Design review of the part shown in the three views and the two pictorial views. Dimensions are in mm from the part's minimum x, y and z. A direction names the side the tool comes from. Round coordinates to 2 decimals unless told otherwise and drop trailing zeros. Write each loop counter-clockwise with the first axis right and the second up, starting at its lowest first coordinate (ties: lowest second). Pieces come first, ordered by that corner, then holes. Notation, with made-up numbers: (60.5, -39.75) -> (119.5, -39.75) arc R9 ccw to (119.5, -33.75) -> close; hole circle Ø11 at (86.25, 29). An arc over 180 degrees is marked (long way). Return JSON: item names as keys, results as strings. Group by question number.
1. Mouldability with a two-part tool opening along Z and no side actions: class the marked faces 1, 2, 3 and 4 as pulls with the +Z half, pulls with the -Z half, needs draft (parallel to the pull), parting line crosses it, or undercut.
2. Take a section at A-A, the plane y = 5. Write out the cut boundary in (x, z).
3. For line 1 along X through (y, z) = (30, 15.25); line 2 along Z through (x, y) = (6.75, 30); line 3 along Y through (x, z) = (18.5, 11), list the stretches that pass through material, from the lowest coordinate up. Write a range as from..to.
4. Take a section at C-C, the plane z = 12.5. Write out the cut boundary in (x, y).
5. Take a section at D-D, the plane x = 33. Write out the cut boundary in (y, z).
6. Tool access review of the marked faces 5, 6, 7 and 8: name each direction out of +Z, -Z, +X, -X, +Y, -Y from which nothing blocks a thin tool from reaching the whole face with its end or side.
7. Take a section at B-B, the plane y = 30. Write out the cut boundary in (x, z).
8. Clearance check with flat-ended pins moving along their axes: P1, Ø5.5, axis at y = 30, z = 12.5, coming from the -X side; P2, Ø5, axis at y = 53.5, z = 11, coming from the -X side; P3, Ø2, axis at x = 58, z = 9.5, coming from the -Y side. State where each tip first meets the part, or that it passes through.
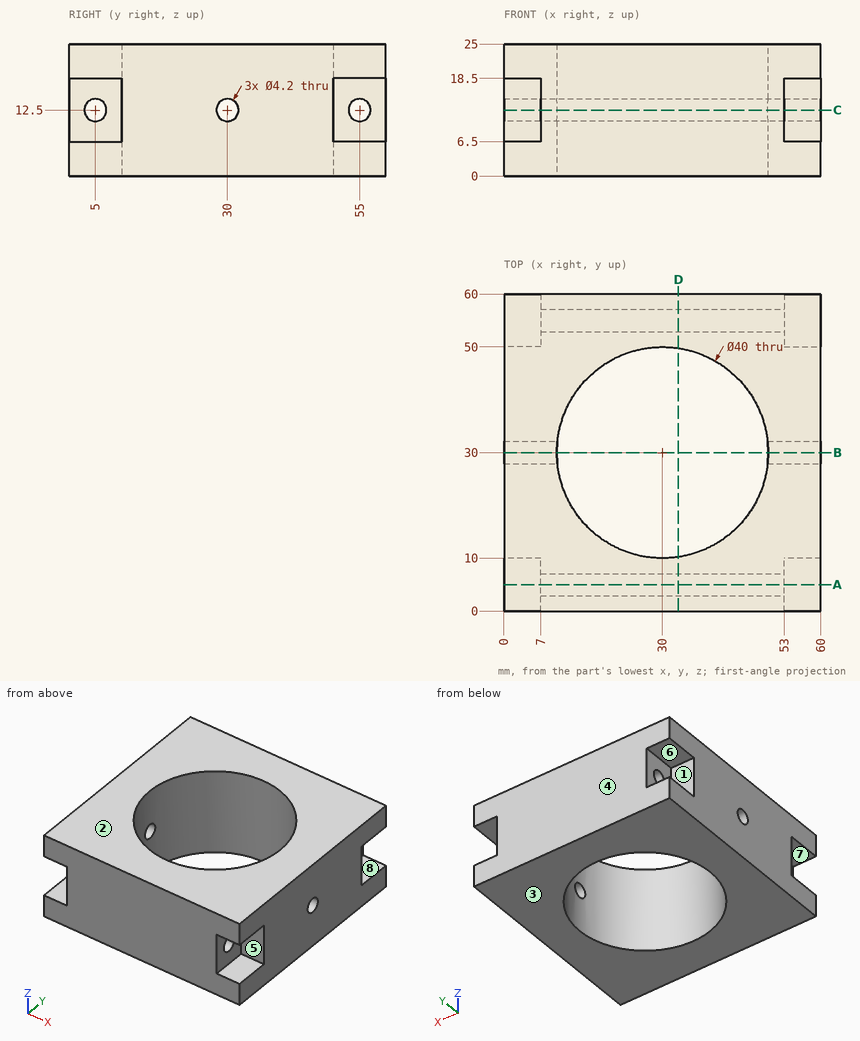
Output:
{
 "1": {"face 1": "undercut", "face 2": "pulls with the +Z half", "face 3": "pulls with the -Z half", "face 4": "needs draft"},
 "2": {"outline": "(0, 0) -> (60, 0) -> (60, 6.5) -> (53, 6.5) -> (53, 10.4) -> (7, 10.4) -> (7, 6.5) -> (0, 6.5) -> close; (0, 18.5) -> (7, 18.5) -> (7, 14.6) -> (53, 14.6) -> (53, 18.5) -> (60, 18.5) -> (60, 25) -> (0, 25) -> close"},
 "3": {"line 1": "x = 0..10, 50..60", "line 2": "z = 0..10.4, 14.6..25", "line 3": "y = 0..3.53, 6.47..13.64, 46.36..53.53, 56.47..60"},
 "4": {"outline": "(0, 10) -> (7, 10) -> (7, 7.1) -> (53, 7.1) -> (53, 10) -> (60, 10) -> (60, 27.9) -> (49.89, 27.9) arc R20 cw to (10.11, 27.9) -> (0, 27.9) -> close; (0, 32.1) -> (10.11, 32.1) arc R20 cw to (49.89, 32.1) -> (60, 32.1) -> (60, 50) -> (53, 50) -> (53, 52.9) -> (7, 52.9) -> (7, 50) -> (0, 50) -> close; (7, 0) -> (53, 0) -> (53, 2.9) -> (7, 2.9) -> close; (7, 57.1) -> (53, 57.1) -> (53, 60) -> (7, 60) -> close"},
 "5": {"outline": "(0, 0) -> (10.23, 0) -> (10.23, 25) -> (0, 25) -> close; (49.77, 0) -> (60, 0) -> (60, 25) -> (49.77, 25) -> close; hole circle Ø4.2 at (5, 12.5); hole circle Ø4.2 at (55, 12.5)"},
 "6": {"face 5": "+X, -Y", "face 6": "-X, +Y", "face 7": "-X, -Y", "face 8": "+X, +Y"},
 "7": {"outline": "(0, 0) -> (10, 0) -> (10, 10.4) -> (0, 10.4) -> close; (0, 14.6) -> (10, 14.6) -> (10, 25) -> (0, 25) -> close; (50, 0) -> (60, 0) -> (60, 10.4) -> (50, 10.4) -> close; (50, 14.6) -> (60, 14.6) -> (60, 25) -> (50, 25) -> close"},
 "8": {"P1": "stops at x = 0", "P2": "stops at x = 7", "P3": "stops at y = 10"}
}
